Could you check a few things on this model? Use its own coordinates, in mm. A direction names the side the tool comes from. Give positions to 0.01 mm unless a question says otherwise; leave off trailing zeros. Loops run counter-clockwise (first coordinate to the right, second up) from the corner with the lowest first, then second, coordinate; pieces in that order, holes last. Notation, with made-up numbers: (85, 44.25) -> (100, 44.25) arc R6 ccw to (100, 49.25) -> close; hole circle Ø9 at (26, -28.5). An arc over 180 degrees is marked (long way). Write item = value, one per line. Start each with the question number.
1) On a 3-axis mill with a long thin cutter (end or side, diameter ignored), from which of +Z, -Z, +X, -X, +Y, -Y can I reach the whole of each face in a straight line? I mean faces 4 (the face through (-25, -28, -2)), 5 (the face through (71, -28, -30)), 6 (the face through (69.856, -27.294, -2.566)), 7 (the face through (2, -26, -23)). Say none if no direction works.
2) I want a section at B-B (z = -35). List the corners of the cut face in (x, y) for me.
3) I want a section at C-C (y = -10). List the corners of the cut face in (x, z) for me, and give its area (3 significant figures).
4) I'm going to push flat-ended pins straight in: pin 1 Ø8 at (x, z) = (55, -29.5) entering from +Y; pin 2 Ø1 at (x, y) = (15, -9) entering from -Z; pin 3 Ø4.5 at (y, z) = (-29.5, -1.5) entering from +X. Where does each tip first touch, or does it pass through?
5) If we mould it in two halves opening along X, with no side actions, what happens to faces 1 (the face through (-69, -25, -6)), 2 (the face through (112.5, -7.3, -3.7)), 3 (the face through (75, 25, -2))? For each: +X half, -X half, draft (parallel to the pull), parting line (faces both ways), or undercut.
6) I want a section at D-D (x = -82.5). List the corners of the cut face in (y, z) for me.
7) I need wall thicknesses on probe 1 along X at (y, z) = (-27.8, -20); probe 2 along Z at (x, y) = (0, -28.6); probe 3 along X at (y, z) = (-27, -35). Which ranges of each line are inside material? Lowest first, please. Write a range as from..to.
8) I want a section at A-A (x = 75). List the corners of the cut face in (y, z) for me.
from build123d import *

# Parameters (mm, degrees)
SKETCH_6_W                       = 225
SKETCH_6_H                       = 60
SM_BASE_FLANGE_1_DEPTH           = 4
SM_EDGE_FLANGE_1_STRIP_W         = 26
SM_EDGE_FLANGE_1_STRIP_H         = 4
SM_EDGE_FLANGE_1_STRIP_CUT_DEPTH = 225
SM_EDGE_FLANGE_1_DEPTH           = 225
CUT_EXTRUDE_2_DEPTH              = 5
HOLE_WIZARD_M81_D                = 9
SKETCH_21_W                      = 52
SKETCH_21_H                      = 17
CUT_EXTRUDE_3_DEPTH              = 10
SKETCH_22_W                      = 50
SKETCH_22_H                      = 16
EXTRUDE_1_DEPTH                  = 4
SKETCH_23_W                      = 21
SKETCH_23_H                      = 5
CUT_EXTRUDE_4_DEPTH              = 10
SKETCH_26_R                      = 4.5
CUT_EXTRUDE_5_DEPTH              = 15
FILLET_1_R                       = 2


# Sheet-metal steps are written as plain solids
with BuildPart() as part:
    # Эскиз6 → Базовая кромка1 (new body)
    with BuildSketch(Plane.XY):
        Rectangle(SKETCH_6_W, SKETCH_6_H)
    extrude(amount=-SM_BASE_FLANGE_1_DEPTH)

    # Ребро-кромка1 strip (across the edge) → Ребро-кромка1 strip cut (cut)
    with BuildSketch(Plane(origin=(112.5, -30, -4), x_dir=(0, 1, 0), z_dir=(-1, 0, 0))):
        with Locations((-4, -2)):
            Rectangle(SM_EDGE_FLANGE_1_STRIP_W, SM_EDGE_FLANGE_1_STRIP_H)
    extrude(amount=SM_EDGE_FLANGE_1_STRIP_CUT_DEPTH, mode=Mode.SUBTRACT)

    # Ребро-кромка1 section (across the edge) → Ребро-кромка1 (add)
    with BuildSketch(Plane(origin=(112.5, -30, -4), x_dir=(0, 1, 0), z_dir=(-1, 0, 0))):
        with BuildLine():
            Line((0, 5), (0, 41))
            Line((0, 41), (4, 41))
            Line((4, 41), (4, 5))
            ThreePointArc((4, 5), (5.464466094, 1.464466094), (9, 0))
            Line((9, 0), (9, -4))
            ThreePointArc((9, -4), (2.636038969, -1.363961031), (0, 5))
        make_face()
    extrude(amount=SM_EDGE_FLANGE_1_DEPTH)

    # Эскиз15 → Вырез-Вытянуть2 (cut)
    with BuildSketch(Plane.XZ.offset(30)):
        Polygon((-112.5, -45), (-112.5, -30), (-30, -30), (-15, -45), align=None)
        Polygon((15, -45), (112.5, -45), (112.5, -30), (30, -30), align=None)
    extrude(amount=-CUT_EXTRUDE_2_DEPTH, mode=Mode.SUBTRACT)

    # Отверстие с зазором M81 (through all)
    with Locations(Plane(origin=(0, -30, 0), x_dir=(-1, 0, 0), z_dir=(0, -1, 0))):
        with Locations((-75, 20), (75, 20), (0, 35)):
            Hole(HOLE_WIZARD_M81_D / 2)

    # Эскиз21 → Вырез-Вытянуть3 (cut)
    with BuildSketch(Plane.XZ.offset(30)):
        with Locations((0, -8.5)):
            Rectangle(SKETCH_21_W, SKETCH_21_H)
    extrude(amount=-CUT_EXTRUDE_3_DEPTH, mode=Mode.SUBTRACT)

    # Эскиз22 → Бобышка-Вытянуть1 (add)
    with BuildSketch(Plane.XY):
        with Locations((0, -28)):
            Rectangle(SKETCH_22_W, SKETCH_22_H)
    extrude(amount=-EXTRUDE_1_DEPTH)

    # Эскиз23 → Вырез-Вытянуть4 (cut)
    with BuildSketch(Plane.XY):
        with Locations((-75, 27.5)):
            Rectangle(SKETCH_23_W, SKETCH_23_H)
        with Locations((75, 27.5)):
            Rectangle(SKETCH_23_W, SKETCH_23_H)
    extrude(amount=-CUT_EXTRUDE_4_DEPTH, mode=Mode.SUBTRACT)

    # Эскиз26 → Вырез-Вытянуть5 (cut)
    with BuildSketch(Plane(origin=(0, 0, -4), x_dir=(-1, 0, 0), z_dir=(0, 0, -1))):
        with Locations((-55, 10)):
            Circle(SKETCH_26_R)
        with Locations((55, 10)):
            Circle(SKETCH_26_R)
        with Locations((0, -10)):
            Circle(SKETCH_26_R)
    extrude(amount=-CUT_EXTRUDE_5_DEPTH, mode=Mode.SUBTRACT)

    # Скругление1
    fillet_1_edges = [part.edges().sort_by_distance(p)[0] for p in [
        (15, -28, -45),
        (-15, -28, -45),
        (-112.5, -28, -30),
        (-30, -28, -30),
        (30, -28, -30),
        (112.5, -28, -30),
        (-112.5, 30, -2),
        (112.5, 30, -2),
    ]]
    fillet(fillet_1_edges, radius=FILLET_1_R)


solid = part.part
Answer list:
q1.face_4 = +Z, -Y
q1.face_5 = -Z, +X, +Y, -Y
q1.face_6 = +Z, +X, -Y
q1.face_7 = -Z, +X, -X, +Y
q2.outline = (-25, -30) -> (-4.5, -30) -> (-4.5, -26) -> (-25, -26) -> close; (4.5, -30) -> (25, -30) -> (25, -26) -> (4.5, -26) -> close
q3.outline = (-112.5, -4) -> (-4.5, -4) -> (-4.5, 0) -> (-112.5, 0) -> close; (4.5, -4) -> (112.5, -4) -> (112.5, 0) -> (4.5, 0) -> close
q3.area = 864 mm^2
q4.pin_1 = -26
q4.pin_2 = -4
q4.pin_3 = 25
q5.face_1 = draft
q5.face_2 = +X half
q5.face_3 = undercut
q6.outline = (-30, -30) -> (-26, -30) -> (-26, -9) arc R5 cw to (-21, -4) -> (25, -4) -> (25, 0) -> (-21, 0) arc R9 ccw to (-30, -9) -> close
q7.probe_1 = -112.5..-79.5, -70.5..70.5, 79.5..112.5
q7.probe_2 = -45..-39.5, -30.5..-17, -4..0
q7.probe_3 = -25..-4.5, 4.5..25
q8.outline = (-30, -30) -> (-26, -30) -> (-26, -24.5) -> (-30, -24.5) -> close; (-30, -15.5) -> (-26, -15.5) -> (-26, -9) arc R5 cw to (-21, -4) -> (25, -4) -> (25, 0) -> (-21, 0) arc R9 ccw to (-30, -9) -> close
